```python
from build123d import *

# Parameters (mm, degrees)
MAINBODY_EXTRUDE_START        = -15
MAINBODY_EXTRUDE_DEPTH        = 30
PIVOTSHAFTHOLE_CUT_DEPTH      = 98.724101428
PIVOTSHAFTHOLE_CUT_DEPTH_BACK = 98.724101428
PIVOTSHAFTHOLE_SKETCH_R       = 2.51


with BuildPart() as part:
    # projectionYz_sketch → mainBody_extrude (new body)
    with BuildSketch(Plane(origin=(0, 0, 0), x_dir=(0, 0, -1), z_dir=(1, 0, 0)).offset(MAINBODY_EXTRUDE_START)):
        Polygon((90, -35), (90, -20), (40, -20), (40, 35), (-40, 35), (-40, -20), (-90, -20), (-90, -35), align=None)
    extrude(amount=MAINBODY_EXTRUDE_DEPTH)

    # pivotShaftHole_sketch → pivotShaftHole_cut (cut, two sides: drawn at the far end of the back side and taken through both)
    with BuildSketch(Plane(origin=(0, 0, 0), x_dir=(0, 0, -1), z_dir=(1, 0, 0)).offset(-PIVOTSHAFTHOLE_CUT_DEPTH_BACK)):
        with Locations((-60, -28)):
            Circle(PIVOTSHAFTHOLE_SKETCH_R)
    extrude(amount=PIVOTSHAFTHOLE_CUT_DEPTH + PIVOTSHAFTHOLE_CUT_DEPTH_BACK, mode=Mode.SUBTRACT)


solid = part.part
```
The listing builds one solid part. Answer for the finished solid, in the listing's coordinates (mm). A direction names the side the tool comes from. Coordinates: 2 decimals unless noted, no trailing zeros. Write each loop counter-clockwise with the first axis right and the second up, starting at its lowest first coordinate (ties: lowest second). Pieces come first, ordered by that corner, then holes. Notation, with made-up numbers: M 65.25,-26.75 L 124.25,-26.75 A17 cw 124.25,-4.75 Z; hole C 4,51.25 d2. An arc over 180 degrees is marked long. Use a Markdown table: item, result. Add a question column.
1. Section A-A (y = -28) is taken. Give the vertices of the cut face in (x, z).
2. Section C-C (x = -6.25) is taken. Give the vertices of the cut face in (y, z).
3. Straight lines are drawn through the part: line 1 along Z through (x, y) = (8.75, -28); line 2 along Y through (x, z) = (-0.5, 60); line 3 along Z through (x, y) = (13.5, -5.5). For each, find the intervals that lie inside material, in ascending order. Write a range as [from, to].
4. Section D-D (y = 19.5) is taken. Give the vertices of the cut face in (x, z), plus the area to 3 significant figures.
5. Which of the six approach directions +Z, -Z, +X, -X, +Y, -Y give full straight-line access (tool end or side, diameter ignored) to faces 1 (the flat face through (0, 8, 40)), 2 (the flat face through (0, 7, -40)), 3 (the flat face through (0, -35, 1))?
6. Given P1, Ø1, axis at x = -3.5, y = 27.5, coming from the +Z side; P2, Ø1.5, axis at x = 3.5, y = -4, coming from the -Z side; P3, Ø8, axis at y = -28, z = 60, coming from the -X side; P4, Ø9, axis at x = 5, z = 63.5, coming from the +Y side, each flat-ended and moving along its own axis, determine where each tip first touches the part or whether it passes through.
7. Section B-B (z = 60) is taken. Give the vertices of the cut face in (x, y), plus the area to 3 significant figures.
Data:
| question | item | result |
|---|---|---|
| 1 | outline | M -15,-90 L 15,-90 L 15,57.49 L -15,57.49 Z; M -15,62.51 L 15,62.51 L 15,90 L -15,90 Z |
| 2 | outline | M -35,-90 L -20,-90 L -20,-40 L 35,-40 L 35,40 L -20,40 L -20,90 L -35,90 Z; hole C -28,60 d5.02 |
| 3 | line 1 | z = [-90, 57.49], [62.51, 90] |
| 3 | line 2 | y = [-35, -30.51], [-25.49, -20] |
| 3 | line 3 | z = [-40, 40] |
| 4 | outline | M -15,-40 L 15,-40 L 15,40 L -15,40 Z |
| 4 | area | 2,400 mm2 |
| 5 | face 1 | +Z, +X, -X, +Y |
| 5 | face 2 | -Z, +X, -X, +Y |
| 5 | face 3 | +Z, -Z, +X, -X, -Y |
| 6 | P1 | stops at z = 40 |
| 6 | P2 | stops at z = -40 |
| 6 | P3 | stops at x = -15 |
| 6 | P4 | stops at y = -20 |
| 7 | outline | M -15,-35 L 15,-35 L 15,-30.51 L -15,-30.51 Z; M -15,-25.49 L 15,-25.49 L 15,-20 L -15,-20 Z |
| 7 | area | 299 mm2 |
